Geometry: final body of the model. Coordinates: model frame, mm. A direction names the side the tool comes from. Round coordinates to 2 decimals unless told otherwise and drop trailing zeros. Put each result on its own line as item: value.
```python
from build123d import *

# Parameters (mm, degrees)
SKETCH1_R           = 2.375
SKETCH1_R_2         = 1.225
SKETCH1_R_3         = 1.125
SKETCH1_W           = 8.25
SKETCH1_H           = 2
SKETCH1_W_2         = 5
SKETCH1_W_3         = 6.000000352
SKETCH1_H_2         = 4
BOSS_EXTRUDE1_DEPTH = 4
SKETCH3_W           = 8
SKETCH3_H           = 4
CUT_EXTRUDE2_DEPTH  = 5
SKETCH4_R           = 2.1
CUT_EXTRUDE3_DEPTH  = 2
SKETCH5_R           = 1.5
BOSS_EXTRUDE2_DEPTH = 1.2


with BuildPart() as part:
    # Sketch1 → Boss-Extrude1 (new body)
    with BuildSketch(Plane.XY):
        with BuildLine():
            Line((-12.978641063, -17.999999648), (-12.978641063, -24))
            Line((-12.978641063, -24), (23.021361236, -24))
            Line((23.021361236, -24), (23.021361236, -17.999999648))
            ThreePointArc((23.021361236, -17.999999648), (33.533081461, -15.187018076), (41.234956591, -7.5))
            ThreePointArc((41.234956591, -7.5), (47.261249953, 9.161168651), (49.306345049, 26.760269155))
            ThreePointArc((49.306345049, 26.760269155), (48.53517536, 46.971383776), (46.226150624, 67.064971353))
            Line((46.226150624, 67.064971353), (30.153849376, 69.095028647))
            Line((30.153849376, 69.095028647), (27.668766331, 75.523635508))
            Line((27.668766331, 75.523635508), (11.471233669, 75.806364492))
            Line((11.471233669, 75.806364492), (8.1, 82.51))
            Line((8.1, 82.51), (-8.1, 82.51))
            Line((-8.1, 82.51), (-15.746235706, 82.281481113))
            Line((-15.746235706, 82.281481113), (-31.943764294, 81.998518887))
            ThreePointArc((-31.943764294, 81.998518887), (-38.536008, 47.204020641), (-37.052658257, 11.821617405))
            ThreePointArc((-37.052658257, 11.821617405), (-29.003702847, -6.308616172), (-12.978641063, -17.999999648))
        make_face()
        with Locations((38.147341743, 11.821617405)):
            Circle(SKETCH1_R, mode=Mode.SUBTRACT)
        with Locations((-27.1, 8.875641236)):
            Circle(SKETCH1_R_2, mode=Mode.SUBTRACT)
        with Locations((-27.1, 16.875641236)):
            Circle(SKETCH1_R_2, mode=Mode.SUBTRACT)
        with Locations((-11.1, 8.875641236)):
            Circle(SKETCH1_R_2, mode=Mode.SUBTRACT)
        with Locations((-11.1, 16.875641236)):
            Circle(SKETCH1_R_2, mode=Mode.SUBTRACT)
        with Locations((-5.25, 80.01)):
            Circle(SKETCH1_R_3, mode=Mode.SUBTRACT)
        with Locations((32.668103408, 66.257595536)):
            Circle(SKETCH1_R_3, mode=Mode.SUBTRACT)
        with Locations((-31.681501662, 43.456405989)):
            Circle(SKETCH1_R, mode=Mode.SUBTRACT)
        with Locations((5.25, 80.01)):
            Circle(SKETCH1_R_3, mode=Mode.SUBTRACT)
        with Locations((5.25, 74.01)):
            Circle(SKETCH1_R_3, mode=Mode.SUBTRACT)
        with Locations((-5.25, 74.01)):
            Circle(SKETCH1_R_3, mode=Mode.SUBTRACT)
        with Locations((-29.050567347, 79.548639007)):
            Circle(SKETCH1_R_3, mode=Mode.SUBTRACT)
        with Locations((-18.552097199, 79.732041708)):
            Circle(SKETCH1_R_3, mode=Mode.SUBTRACT)
        with Locations((-28.945766522, 73.549554345)):
            Circle(SKETCH1_R_3, mode=Mode.SUBTRACT)
        with Locations((-18.447296374, 73.732957046)):
            Circle(SKETCH1_R_3, mode=Mode.SUBTRACT)
        with Locations((24.670854945, 67.074669457)):
            Circle(SKETCH1_R_3, mode=Mode.SUBTRACT)
        with Locations((14.172454146, 67.257919725)):
            Circle(SKETCH1_R_3, mode=Mode.SUBTRACT)
        with Locations((24.775569383, 73.073755628)):
            Circle(SKETCH1_R_3, mode=Mode.SUBTRACT)
        with Locations((14.277168584, 73.257005896)):
            Circle(SKETCH1_R_3, mode=Mode.SUBTRACT)
        with Locations((31.916230336, 60.30489137)):
            Circle(SKETCH1_R_3, mode=Mode.SUBTRACT)
        with Locations((43.457736871, 64.89478048)):
            Circle(SKETCH1_R_3, mode=Mode.SUBTRACT)
        with Locations((42.705863799, 58.942076315)):
            Circle(SKETCH1_R_3, mode=Mode.SUBTRACT)
        with Locations((0, 77.51)):
            Rectangle(SKETCH1_W, SKETCH1_H, mode=Mode.SUBTRACT)
        Polygon((-10.203, 23.9877015), (-9.6615, 28.865490815), (-23.703732608, 30.424366869), (-23.262390208, 34.399944423), (-31.213545315, 35.282629224), (-31.654887716, 31.30705167), (-34.636570881, 31.63805847), (-35.178070881, 26.760269155), (-32.196387716, 26.429262355), (-32.637730116, 22.453684801), (-24.686575009, 21.571), (-24.245232608, 25.546577554), align=None, mode=Mode.SUBTRACT)
        with BuildLine():
            Line((10.358817838, 63.151218734), (10.358817838, 60.151218734))
            Line((10.358817838, 60.151218734), (8.358817838, 60.151218734))
            ThreePointArc((8.358817838, 60.151218734), (-5.478579327, 61.651218734), (8.358817838, 63.151218734))
            Line((8.358817838, 63.151218734), (10.358817838, 63.151218734))
        make_face(mode=Mode.SUBTRACT)
        with Locations((35.147341743, 56.321617405)):
            Rectangle(SKETCH1_W_2, SKETCH1_H, mode=Mode.SUBTRACT)
        with BuildLine():
            Line((-17.84156291, 63.151218734), (-15.84156291, 63.151218734))
            Line((-15.84156291, 63.151218734), (-15.84156291, 60.151218734))
            Line((-15.84156291, 60.151218734), (-17.84156291, 60.151218734))
            ThreePointArc((-17.84156291, 60.151218734), (-31.678960076, 61.651218734), (-17.84156291, 63.151218734))
        make_face(mode=Mode.SUBTRACT)
        Polygon((-28.274482275, 78.062008978), (-19.275783292, 78.219211472), (-19.240849684, 76.219516585), (-28.239548667, 76.06231409), align=None, mode=Mode.SUBTRACT)
        with Locations((17.86306514, 56.321617405)):
            Rectangle(SKETCH1_W_2, SKETCH1_H, mode=Mode.SUBTRACT)
        with Locations((-0.478579327, 71.151218734)):
            Rectangle(SKETCH1_W_2, SKETCH1_H, mode=Mode.SUBTRACT)
        Polygon((15.375818632, 71.737600396), (15.340913819, 69.737905006), (23.589657304, 69.593922653), (23.624562117, 71.593618043), align=None, mode=Mode.SUBTRACT)
        with BuildLine():
            Line((8.025667975, 48.321617405), (6.025667975, 48.321617405))
            Line((6.025667975, 48.321617405), (6.025667975, 45.321617405))
            Line((6.025667975, 45.321617405), (8.025667975, 45.321617405))
            ThreePointArc((8.025667975, 45.321617405), (21.86306514, 46.821617405), (8.025667975, 48.321617405))
        make_face(mode=Mode.SUBTRACT)
        Polygon((42.153636572, 63.54758064), (33.223865999, 64.675480473), (32.973241642, 62.691245751), (41.903012214, 61.563345918), align=None, mode=Mode.SUBTRACT)
        with BuildLine():
            Line((29.309944577, 45.321617405), (31.309944577, 45.321617405))
            ThreePointArc((31.309944577, 45.321617405), (45.147341743, 46.821617405), (31.309944577, 48.321617405))
            Line((31.309944577, 48.321617405), (29.309944577, 48.321617405))
            Line((29.309944577, 48.321617405), (29.309944577, 45.321617405))
        make_face(mode=Mode.SUBTRACT)
        with Locations((-22.678960076, 71.151218734)):
            Rectangle(SKETCH1_W_2, SKETCH1_H, mode=Mode.SUBTRACT)
        Polygon((-4, -2.5), (0, -2.5), (0, 0), (12, 0), (12, -2.5), (16, -2.5), (16, -12.5), (12, -12.5), (12, -15), (0, -15), (0, -12.5), (-4, -12.5), align=None, mode=Mode.SUBTRACT)
        Polygon((0, 23.56093555), (-3, 23.56093555), (-4.5, 20.962859339), (-3, 18.364783128), (0, 18.364783128), (1.5, 20.962859339), align=None, mode=Mode.SUBTRACT)
        with Locations((-2.036620161, 8.717005814)):
            Rectangle(SKETCH1_W_3, SKETCH1_H_2, mode=Mode.SUBTRACT)
        with Locations((-2.036620161, 33.335566927)):
            Rectangle(SKETCH1_W_3, SKETCH1_H_2, mode=Mode.SUBTRACT)
    extrude(amount=BOSS_EXTRUDE1_DEPTH)

    # Sketch3 → Cut-Extrude2 (cut, through all)
    with BuildSketch(Plane(origin=(0, 0, 0), x_dir=(-1, 0, 0), z_dir=(0, 0, -1))):
        with Locations((-28.271360086, -8)):
            Rectangle(SKETCH3_W, SKETCH3_H)
        with Locations((18.228639914, -8)):
            Rectangle(SKETCH3_W, SKETCH3_H)
    extrude(amount=-CUT_EXTRUDE2_DEPTH, mode=Mode.SUBTRACT)

    # Sketch4 → Cut-Extrude3 (cut)
    with BuildSketch(Plane(origin=(0, 0, 0), x_dir=(-1, 0, 0), z_dir=(0, 0, -1))):
        with Locations((27.1, 16.875641236)):
            Circle(SKETCH4_R)
        with Locations((27.1, 8.875641236)):
            Circle(SKETCH4_R)
        with Locations((11.1, 8.875641236)):
            Circle(SKETCH4_R)
        with Locations((11.1, 16.875641236)):
            Circle(SKETCH4_R)
    extrude(amount=-CUT_EXTRUDE3_DEPTH, mode=Mode.SUBTRACT)

    # Sketch5 → Boss-Extrude2 (add)
    with BuildSketch(Plane.XY.offset(4)):
        Polygon((-3.018844903, 18.391695962), (-0.018844903, 18.391695962), (1.481155097, 20.989772174), (-0.018844903, 23.587848385), (-3.018844903, 23.587848385), (-4.518844903, 20.989772174), align=None)
        with Locations((-1.518844903, 20.989772174)):
            Circle(SKETCH5_R, mode=Mode.SUBTRACT)
    extrude(amount=-BOSS_EXTRUDE2_DEPTH)


solid = part.part
```
1. Contact query for flat-ended pins moving along their axis: P1, Ø6.5, axis at x = -27.1, y = 16.88, coming from the -Z side; P2, Ø0.6, axis at y = 56, z = 1.5, coming from the +X side; P3, Ø3, axis at x = -27.1, y = 8.88, coming from the -Z side; P4, Ø1, axis at x = -16.5, z = 2, coming from the -Y side. Output: stop coordinate, or through.
Ans:
P1: z = 0
P2: x = 47.72
P3: z = 2
P4: y = -16.68
2. Draft query along X for faces 1 (the face through (-22.229, -8, 2)), 2 (the face through (-23, 70.151, 2)). Return one class per face: +X half, -X half, draft (parallel to the pull), parting line (faces both ways), or undercut.
Ans:
face 1: undercut
face 2: undercut
3. Cut plane A-A on z = 1.25. State how many separate pieces and enclosed holes the cut face has, and give its area (3 significant figures).
Ans:
separate pieces: 1
enclosed holes: 41
area: 6,490 mm²
4. Material intervals for probe 1 along Y at (x, z) = (17.5, 1.4); probe 2 along X at (y, z) = (18, 1.05); probe 3 along X at (y, z) = (33, 0.4), sorted ascending.
Ans:
probe 1: -24 to 40.34, 53.31 to 55.32, 57.32 to 69.7, 71.7 to 75.7
probe 2: -37.9 to -28.87, -25.33 to -12.87, -9.33 to 48.8
probe 3: -38.92 to -31.47, -23.42 to -5.04, 0.96 to 49.23
5. Set-up query: faces 3 (the face through (-10.645, 14.826, 0.986)), 4 (the face through (-34.904, 29.233, 1.972)). Return all of +Z, -Z, +X, -X, +Y, -Y with unobstructed straight access to the full face (end or side cutting, diameter ignored); none if empty.
Ans:
face 3: -Z
face 4: +Z, -Z
